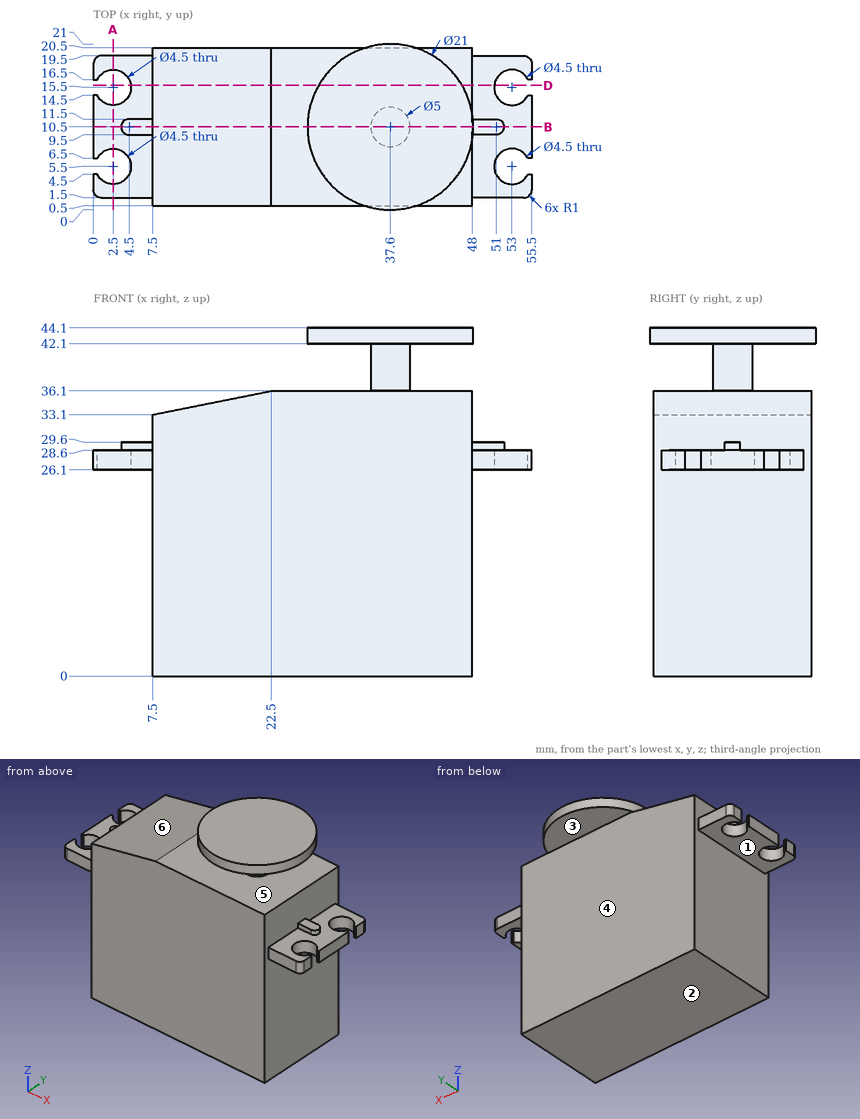
Check sheet for the drawn part. Datum: minimum x, y, z corner. Units: mm. A direction names the side the tool comes from. Give positions to 0.01 mm unless a question says otherwise; leave off trailing zeros. Order: outer loops, then holes, each group sorted by start corner. A loop starts at its lowest first (then second) coordinate and runs counter-clockwise, first axis right, second up. Notation, with made-up numbers: (50.5, -16.75) - (61.5, -16.75) arc R18 cw to (61.5, -11.75) - close; hole circle Ø1 at (-12, 67.25). An arc over 180 degrees is marked (long way). Answer as a JSON object with one key per item and string values.
(1) Tool access check on the marked faces 1, 2 and 3. Record the directions out of +Z, -Z, +X, -X, +Y, -Y that give a thin tool (end or side, any length) a straight path to the whole face; none if there is none.
Report:
{"face 1": "-Z, -X, +Y, -Y", "face 2": "-Z, +X, -X, +Y, -Y", "face 3": "none"}
(2) Cross-section at D-D (y = 15.75). Record the cut outline in (x, z).
Report:
{"outline": "(4.74, 26.1) - (7.5, 26.1) - (7.5, 0) - (48, 0) - (48, 26.1) - (50.76, 26.1) - (50.76, 28.6) - (48, 28.6) - (48, 36.1) - (22.5, 36.1) - (7.5, 33.1) - (7.5, 28.6) - (4.74, 28.6) - close; (28.51, 42.1) - (46.69, 42.1) - (46.69, 44.1) - (28.51, 44.1) - close"}
(3) Material ranges on line 1 (Y direction, x = 53, z = 27.75); line 2 (Z direction, x = 38, y = 2.25); line 3 (Y direction, x = 33.5, z = 7), recorded low to high.
Report:
{"line 1": "1.5 to 3.25, 7.75 to 13.25, 17.75 to 19.5", "line 2": "0 to 36.1, 42.1 to 44.1", "line 3": "0.5 to 20.5"}
(4) Depth check by flat-ended pin: pin 1 Ø6 at (y, z) = (13.5, 19.5) entering from -X; pin 2 Ø3 at (y, z) = (11, 34.5) entering from +X; pin 3 Ø1 at (x, y) = (5, 10.5) entering from +Z; pin 4 Ø2.5 at (x, y) = (53, 5.5) entering from -Z. Enter the tip coordinate at first touch or a pass-through.
Report:
{"pin 1": "x = 7.5", "pin 2": "x = 48", "pin 3": "z = 29.6", "pin 4": "through"}
(5) Cross-section at A-A (x = 2.5). Record the cut outline in (y, z).
Report:
{"outline": "(1.5, 26.1) - (3.25, 26.1) - (3.25, 28.6) - (1.5, 28.6) - close; (7.75, 26.1) - (13.25, 26.1) - (13.25, 28.6) - (7.75, 28.6) - close; (17.75, 26.1) - (19.5, 26.1) - (19.5, 28.6) - (17.75, 28.6) - close"}
(6) Draft check along Z on the marked faces 4, 5 and 6. Enter one of: released by +Z, released by -Z, zero draft, split by the parting line, or undercut.
Report:
{"face 4": "zero draft", "face 5": "undercut", "face 6": "released by +Z"}
(7) Cross-section at B-B (y = 10.5). Record the cut outline in (x, z), then the cut area to 3 significant figures.
Report:
{"outline": "(0, 26.1) - (7.5, 26.1) - (7.5, 0) - (48, 0) - (48, 26.1) - (55.5, 26.1) - (55.5, 28.6) - (52, 28.6) - (52, 29.6) - (48, 29.6) - (48, 36.1) - (40.1, 36.1) - (40.1, 42.1) - (48.1, 42.1) - (48.1, 44.1) - (27.1, 44.1) - (27.1, 42.1) - (35.1, 42.1) - (35.1, 36.1) - (22.5, 36.1) - (7.5, 33.1) - (7.5, 29.6) - (3.5, 29.6) - (3.5, 28.6) - (0, 28.6) - close", "area": "1,560 mm^2"}
